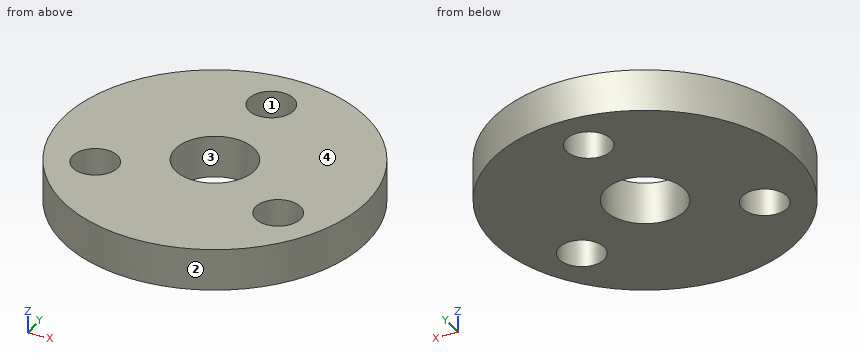
from build123d import *

# Parameters (mm, degrees)
SKETCH1_R           = 11.5
SKETCH1_R_2         = 3
SKETCH1_R_3         = 1.7
BOSS_EXTRUDE1_DEPTH = 3.175


with BuildPart() as part:
    # Sketch1 → Boss-Extrude1 (new body)
    with BuildSketch(Plane.XY):
        with Locations((10.103629711, -10.110058712)):
            Circle(SKETCH1_R)
        with Locations((10.103629711, -10.110058712)):
            Circle(SKETCH1_R_2, mode=Mode.SUBTRACT)
        with Locations((3.175426481, -14.110058712)):
            Circle(SKETCH1_R_3, mode=Mode.SUBTRACT)
        with Locations((17.031832941, -14.110058712)):
            Circle(SKETCH1_R_3, mode=Mode.SUBTRACT)
        with Locations((10.103629711, -2.110058712)):
            Circle(SKETCH1_R_3, mode=Mode.SUBTRACT)
    extrude(amount=BOSS_EXTRUDE1_DEPTH)


solid = part.part
The model under review builds one solid part; all positions refer to its coordinate system, in mm. Face numbers are marked on the shaded views. Give positions to 0.01 mm unless a question says otherwise; leave off trailing zeros. Order: outer loops, then holes, each group sorted by start corner. A loop starts at its lowest first (then second) coordinate and runs counter-clockwise, first axis right, second up. Notation, with made-up numbers: (5.5, -21) -> (41.5, -21) arc R34 cw to (41.5, 13) -> close; hole circle Ø5 at (78.25, -32.75). An arc over 180 degrees is marked (long way). Write item = value, one per line. Start each with the question number.
(1) Take a section at D-D (z = 2.7). Write out the cut boundary in (x, y), plus the area to 3 significant figures.
(2) For pin 1 Ø1 at (y, z) = (-15.5, 0.5) entering from -X; pin 2 Ø3 at (x, y) = (6.5, -3.5) entering from -Z, all flat-tipped, find the tip position at first contact; note any pin that passes through.
(3) Take a section at B-B (x = 2). Write out the cut boundary in (y, z) (3 decimals).
(4) Take a section at C-C (y = -15). Write out the cut boundary in (x, z) (3 decimals), plus the area to 3 significant figures.
(5) Take a section at A-A (y = -11.25). Write out the cut boundary in (x, z) (3 decimals), plus the area to 3 significant figures.
(6) Draft analysis for pull direction Y (two halves, no side actions). For the marked faces 1, 2, 3 and 4, state which applies: +Y half, -Y half, draft (parallel to the pull), parting line (faces both ways), or undercut.
(7) For L1, parallel to X at y = -15.5, z = 3; L2, parallel to Y at x = 11.25, z = 2.85; L3, parallel to X at y = -14, z = 2.55, list the stretches that pass through material, from the lowest coordinate up. Write a range as from..to.
Returned:
q1.outline = circle Ø23 at (10.1, -10.11); hole circle Ø3.4 at (3.18, -14.11); hole circle Ø6 at (10.1, -10.11); hole circle Ø3.4 at (10.1, -2.11); hole circle Ø3.4 at (17.03, -14.11)
q1.area = 360 mm²
q2.pin_1 = -0.3
q2.pin_2 = 0
q3.outline = (-18.27, 0) -> (-15.338, 0) -> (-15.338, 3.175) -> (-18.27, 3.175) -> close; (-12.882, 0) -> (-1.95, 0) -> (-1.95, 3.175) -> (-12.882, 3.175) -> close
q4.outline = (-0.305, 0) -> (1.727, 0) -> (1.727, 3.175) -> (-0.305, 3.175) -> close; (4.624, 0) -> (15.583, 0) -> (15.583, 3.175) -> (4.624, 3.175) -> close; (18.48, 0) -> (20.512, 0) -> (20.512, 3.175) -> (18.48, 3.175) -> close
q4.area = 47.7 mm²
q5.outline = (-1.34, 0) -> (7.329, 0) -> (7.329, 3.175) -> (-1.34, 3.175) -> close; (12.879, 0) -> (21.547, 0) -> (21.547, 3.175) -> (12.879, 3.175) -> close
q5.area = 55.0 mm²
q6.face_1 = undercut
q6.face_2 = parting line
q6.face_3 = undercut
q6.face_4 = draft
q7.L1 = -0.06..2.2, 4.15..16.05, 18.01..20.26
q7.L2 = -21.55..-12.88, -7.34..-3.37, -0.85..1.33
q7.L3 = -0.72..1.48, 4.87..15.34, 18.73..20.93
